```python
from build123d import *

# Parameters (mm, degrees)
BOSS_EXTRUDE1_DEPTH = 2.54
BOSS_EXTRUDE4_DEPTH = 20.32
SKETCH3_W           = 31.75
SKETCH3_H           = 16.51
CUT_EXTRUDE1_DEPTH  = 2.54


with BuildPart() as part:
    # Sketch1 → Boss-Extrude1 (new body)
    with BuildSketch(Plane(origin=(0, 0, 0), x_dir=(1, 0, 0), z_dir=(0, 1, 0))):
        with BuildLine():
            Line((0, 0), (31.75, 0))
            Line((31.75, 0), (31.75, 26.649569904))
            ThreePointArc((31.75, 26.649569904), (15.875, 31.75), (0, 26.649569904))
            Line((0, 26.649569904), (0, 0))
        make_face()
    extrude(amount=BOSS_EXTRUDE1_DEPTH)

    # Sketch2 → Boss-Extrude4 (add)
    with BuildSketch(Plane(origin=(0, 2.54, 0), x_dir=(1, 0, 0), z_dir=(0, 1, 0))):
        with BuildLine():
            Line((31.75, 22.059647753), (31.75, 26.649569904))
            ThreePointArc((31.75, 26.649569904), (15.875, 31.75), (0, 26.649569904))
            Line((0, 26.649569904), (0, 22.059647753))
            ThreePointArc((0, 22.059647753), (15.875, 27.178), (31.75, 22.059647753))
        make_face()
        with BuildLine():
            Line((2.54, 26.911706478), (2.54, 24.951669261))
            ThreePointArc((2.54, 24.951669261), (15.875, 28.448), (29.21, 24.951669261))
            Line((29.21, 24.951669261), (29.21, 27.054735))
            ThreePointArc((29.21, 27.054735), (15.856249221, 30.479609179), (2.54, 26.911706478))
        make_face(mode=Mode.SUBTRACT)
    extrude(amount=BOSS_EXTRUDE4_DEPTH)

    # Sketch3 → Cut-Extrude1 (cut)
    with BuildSketch(Plane(origin=(0, 2.54, 0), x_dir=(1, 0, 0), z_dir=(0, 1, 0))):
        with Locations((15.875, 8.255)):
            Rectangle(SKETCH3_W, SKETCH3_H)
    extrude(amount=-CUT_EXTRUDE1_DEPTH, mode=Mode.SUBTRACT)


solid = part.part
```
Geometry: final body of the model. Coordinates: model frame, mm. A direction names the side the tool comes from. Round coordinates to 2 decimals unless told otherwise and drop trailing zeros. Loops run counter-clockwise (first coordinate to the right, second up) from the corner with the lowest first, then second, coordinate; pieces in that order, holes last. Notation, with made-up numbers: (63.25, 1.5) -> (113.25, 1.5) arc R16 cw to (113.25, 28.5) -> close; hole circle Ø6 at (5.25, 32.25). An arc over 180 degrees is marked (long way). Use one line per item in the form item = value. Start each with the question number.
1) First-contact query: P1, Ø1.5, axis at x = 9, y = 12.5, coming from the +Z side; P2, Ø3, axis at x = 9.5, y = 5, coming from the +Z side; P3, Ø3, axis at x = 22, z = -20.5, coming from the +Y side. Flat tips, straight axial feed; report the tip coordinate or a pass-through.
2) Section D-D on x = 20.5. Output: boundary loops of the cut face in (y, z), then the cut area to 3 significant figures.
3) Access query for faces 4 (the flat face through (2.54, 13, -26)), 5 (the flat face through (16, 0, -24)), 6 (the flat face through (16, 2.54, -21)). Directions: +Z, -Z, +X, -X, +Y, -Y. A direction counts if a zero-diameter tool reaches every point of the face in a straight line with its end or side. Return the directions, or none.
4) Section B-B on x = 7. Output: boundary loops of the cut face in (y, z).
5) Draft query along X for faces 1 (the flat face through (0, 11, -24)), 2 (the flat face through (16, 1, -16.51)), 3 (the flat face through (29.21, 13, -26)). Return one class per face: released by +X, released by -X, zero draft, split by the parting line, or undercut.
6) Section A-A on y = 10.5. Output: boundary loops of the cut face in (x, z) (3 decimals).
7) Section C-C on z = -26. Output: boundary loops of the cut face in (x, y), then the cut area to 3 significant figures.
8) Line query: L1, parallel to X at y = 9.5, z = -22.5; L2, parallel to Z at x = 11, y = 4.25; L3, parallel to Z at x = 27.5, y = 20.75. Output: solid intervals per line, ascending.
Response:
q1.P1 = -26.09
q1.P2 = -26.01
q1.P3 = 2.54
q2.outline = (0, -31.35) -> (22.86, -31.35) -> (22.86, -30.11) -> (2.54, -30.11) -> (2.54, -28.05) -> (22.86, -28.05) -> (22.86, -26.78) -> (2.54, -26.78) -> (2.54, -16.51) -> (0, -16.51) -> close
q2.area = 88.9 mm^2
q3.face_4 = +Y
q3.face_5 = +Z, -Z, +X, -X, -Y
q3.face_6 = +Z, +Y
q4.outline = (0, -30.26) -> (22.86, -30.26) -> (22.86, -28.95) -> (2.54, -28.95) -> (2.54, -26.96) -> (22.86, -26.96) -> (22.86, -25.69) -> (2.54, -25.69) -> (2.54, -16.51) -> (0, -16.51) -> close
q5.face_1 = released by -X
q5.face_2 = zero draft
q5.face_3 = undercut
q6.outline = (0, -26.65) arc R27.256 ccw to (31.75, -26.65) -> (31.75, -22.06) arc R27.178 cw to (0, -22.06) -> close; hole (2.54, -26.912) arc R27.178 ccw to (29.21, -27.055) -> (29.21, -24.952) arc R27.178 cw to (2.54, -24.952) -> close
q7.outline = (0, 0) -> (31.75, 0) -> (31.75, 22.86) -> (29.21, 22.86) -> (29.21, 2.54) -> (27.15, 2.54) -> (27.15, 22.86) -> (23.79, 22.86) -> (23.79, 2.54) -> (7.96, 2.54) -> (7.96, 22.86) -> (4.6, 22.86) -> (4.6, 2.54) -> (2.54, 2.54) -> (2.54, 22.86) -> (0, 22.86) -> close
q7.area = 320 mm^2
q8.L1 = 0 to 0.63, 31.12 to 31.75
q8.L2 = -31.31 to -30.02, -28.01 to -26.74
q8.L3 = -29.15 to -27.93, -25.84 to -24.57
